```python
from build123d import *

# Parameters (mm, degrees)
SKETCH1_R           = 1.5
BOSS_EXTRUDE1_DEPTH = 4


with BuildPart() as part:
    # Sketch1 → Boss-Extrude1 (new body)
    with BuildSketch(Plane.XY):
        with BuildLine():
            Line((14.488514014, 22.965384222), (14.488514014, 47.965384222))
            Line((14.488514014, 47.965384222), (7.988514014, 47.965384222))
            Line((7.988514014, 47.965384222), (7.988514014, 22.965384222))
            Line((7.988514014, 22.965384222), (6.488514014, 22.965384222))
            Line((6.488514014, 22.965384222), (0.12000074, 3.87380986))
            ThreePointArc((0.12000074, 3.87380986), (2.018608705, 0.156496466), (5.794859705, 1.93499568))
            Line((5.794859705, 1.93499568), (14.488514014, 22.965384222))
        make_face()
        with Locations((2.988514014, 2.995384222)):
            Circle(SKETCH1_R, mode=Mode.SUBTRACT)
        with Locations((8.988514014, 19.965384222)):
            Circle(SKETCH1_R, mode=Mode.SUBTRACT)
    extrude(amount=BOSS_EXTRUDE1_DEPTH)


solid = part.part
```
Model file for the job. Use its own axes, mm. A direction names the side the tool comes from. Round coordinates to 2 decimals unless told otherwise and drop trailing zeros. Write each loop counter-clockwise with the first axis right and the second up, starting at its lowest first coordinate (ties: lowest second). Pieces come first, ordered by that corner, then holes. Notation, with made-up numbers: (-10.5, -4.75) - (-4.5, -4.75) arc R28 ccw to (-4.5, 33.25) - close; hole circle Ø10 at (-6, -19.75). An arc over 180 degrees is marked (long way). One line per item, written item: value.
(1) Drop flat-ended pins along their axis: P1, Ø2, axis at y = 38.5, z = 1.5, coming from the -X side; P2, Ø0.8, axis at x = 7, z = 2.5, coming from the +Y side. Give the stop position or say it passes through.
Values follow:
P1: stops at x = 7.99
P2: stops at y = 22.97
(2) Cut at A-A, the plane x = 9.25. Give the cut face in (y, z), plus the area to 3 significant figures.
Values follow:
outline: (10.29, 0) - (18.49, 0) - (18.49, 4) - (10.29, 4) - close; (21.44, 0) - (47.97, 0) - (47.97, 4) - (21.44, 4) - close
area: 139 mm²
(3) Two-plate mould, pull along X, no slides. Class faces 1 (the flat face through (14.489, 35, 2)), 2 (the cylindrical face through (1.49, 3.06, 1.97)), 3 (the cylindrical face through (1.958, 0.178, 1.972)): pulls with the +X half, pulls with the -X half, needs draft (parallel to the pull), parting line crosses it, or undercut.
Values follow:
face 1: pulls with the +X half
face 2: undercut
face 3: parting line crosses it
(4) Cut at C-C, the plane y = 38.5. Give the cut face in (x, z), plus the area to 3 significant figures.
Values follow:
outline: (7.99, 0) - (14.49, 0) - (14.49, 4) - (7.99, 4) - close
area: 26.0 mm²
(5) Cut at B-B, the plane z = 1.95. Give the cut face in (x, y) (3 decimals).
Values follow:
outline: (0.12, 3.874) arc R3 ccw to (5.795, 1.935) - (14.489, 22.965) - (14.489, 47.965) - (7.989, 47.965) - (7.989, 22.965) - (6.489, 22.965) - close; hole circle Ø3 at (2.989, 2.995); hole circle Ø3 at (8.989, 19.965)
(6) Cut at D-D, the plane x = 13.5. Give the cut face in (y, z).
Values follow:
outline: (20.57, 0) - (47.97, 0) - (47.97, 4) - (20.57, 4) - close
(7) 3-axis set-ups, long thin cutter, end or side, ignore diameter. For faces 4 (the flat face through (11, 47.965, 2)), 5 (the flat face through (7.989, 36, 2)): which of +Z, -Z, +X, -X, +Y, -Y reach the whole face in a straight line?
Values follow:
face 4: +Z, -Z, +X, -X, +Y
face 5: +Z, -Z, -X, +Y
(8) Wall check: probe 1 along X at (y, z) = (43, 1.4); probe 2 along X at (y, z) = (21, 0.3); probe 3 along Y at (x, z) = (8.75, 3.4). Give the ranges that are in metal, low to high.
Values follow:
probe 1: x = 7.99 to 14.49
probe 2: x = 5.83 to 7.9, 10.07 to 13.68
probe 3: y = 9.08 to 18.48, 21.45 to 47.97
